Check sheet for the drawn part. Datum: minimum x, y, z corner. Units: mm. A direction names the side the tool comes from. Coordinates: 2 decimals unless noted, no trailing zeros. Loops run counter-clockwise (first coordinate to the right, second up) from the corner with the lowest first, then second, coordinate; pieces in that order, holes last. Notation, with made-up numbers: (-2, -10) -> (26, -10) arc R8 cw to (26, 0) -> close; hole circle Ø10 at (29, 18.25). An arc over 180 degrees is marked (long way). Use CSV: the item, a comma, the result in double quotes. Start each with the question number.
1. Sectioned sample at C-C, the plane x = 4.25. Record the cut outline in (y, z).
2. Thickness scan on L1, parallel to Z at x = 4.05, y = 2.25; L2, parallel to X at y = 0.5, z = 4.7. Record the ranges inside material, lowest first.
3. Gauge pin test, flat ends, axial feed: pin 1 (0.6 mm diameter, centred on y = 3, z = 3.5, fed in from -X); pin 2 (0.6 mm diameter, centred on x = 2, z = 4.5, fed in from -Y); pin 3 (0.6 mm diameter, centred on x = 2.5, z = 4, fed in from +Y). Record the tip position at first contact, or that the pin passes through.
4. Sectioned sample at A-A, the plane x = 2.9. Record the cut outline in (y, z).
5. Sectioned sample at D-D, the plane z = 3.65. Record the cut outline in (x, y), and give its area (3 significant figures).
6. Set-up check for the marked faces 1, 2 and 3: record each of +Z, -Z, +X, -X, +Y, -Y from which the full face is reachable in a straight line by a thin tool's end or side.
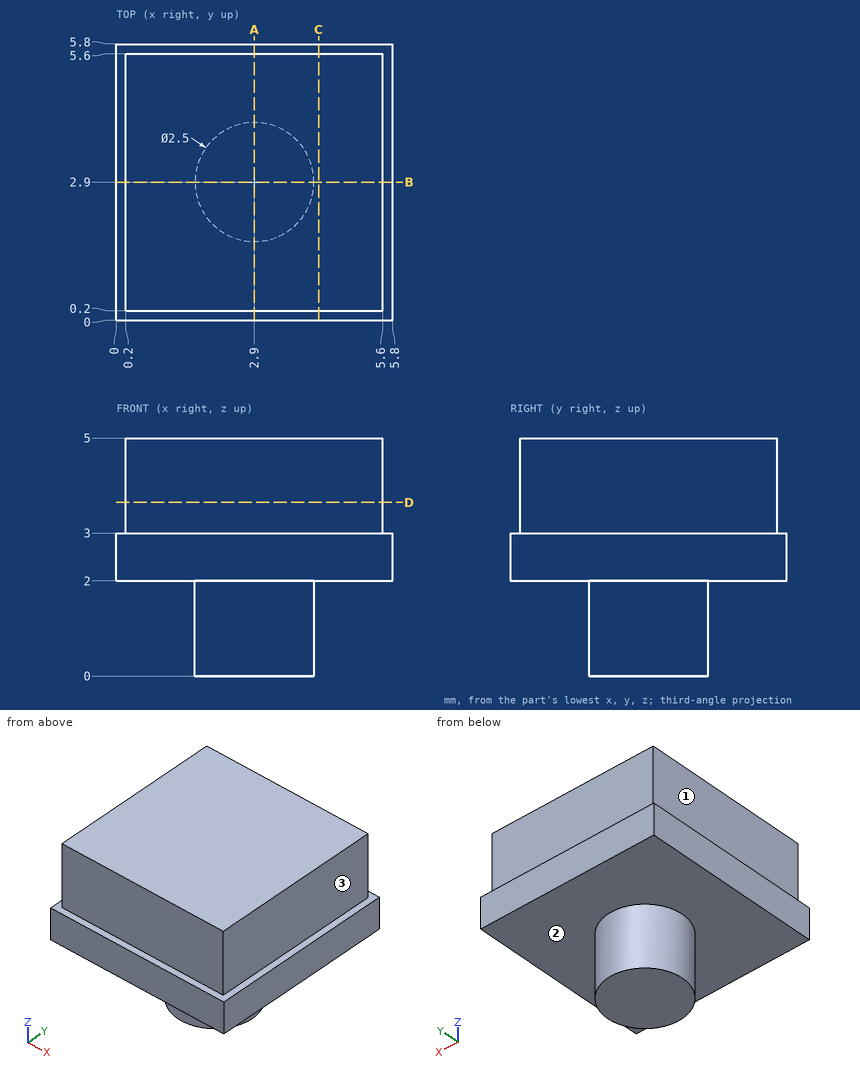
Completed:
1,outline,"(0, 2) -> (5.8, 2) -> (5.8, 3) -> (5.6, 3) -> (5.6, 5) -> (0.2, 5) -> (0.2, 3) -> (0, 3) -> close"
2,L1,"2 to 5"
2,L2,"0.2 to 5.6"
3,pin 1,"x = 0.2"
3,pin 2,"y = 0.2"
3,pin 3,"y = 5.6"
4,outline,"(0, 2) -> (1.65, 2) -> (1.65, 0) -> (4.15, 0) -> (4.15, 2) -> (5.8, 2) -> (5.8, 3) -> (5.6, 3) -> (5.6, 5) -> (0.2, 5) -> (0.2, 3) -> (0, 3) -> close"
5,outline,"(0.2, 0.2) -> (5.6, 0.2) -> (5.6, 5.6) -> (0.2, 5.6) -> close"
5,area,"29.2 mm²"
6,face 1,"+Z, -X, +Y, -Y"
6,face 2,"-Z"
6,face 3,"+Z, +X, +Y, -Y"
